from build123d import *

# Parameters (mm, degrees)
SKETCH_1_R          = 5.5
EXTRUDE_1_DEPTH     = 1
EXTRUDE_2_DEPTH     = 3
CUT_EXTRUDE_2_REACH = 8
SKETCH_9_R          = 2.5
CHAMFER_1_SIZE      = 0.3


with BuildPart() as part:
    # Эскиз1 → Бобышка-Вытянуть1 (new body)
    with BuildSketch(Plane.XY):
        Circle(SKETCH_1_R)
    extrude(amount=EXTRUDE_1_DEPTH)

    # Эскиз3 → Бобышка-Вытянуть2 (add)
    with BuildSketch(Plane.XY.offset(1)):
        Polygon((2.608163285, 3.811930956), (-1.997147402, 4.16470114), (-4.605310688, 0.352770185), (-2.608163285, -3.811930956), (1.997147402, -4.16470114), (4.605310688, -0.352770185), align=None)
    extrude(amount=EXTRUDE_2_DEPTH)

    # Эскиз5 → Вырез-Повернуть3 (revolve, cut)
    with BuildSketch(Plane(origin=(0, 0, 0), x_dir=(-0.997079012, 0.076376985, 0), z_dir=(-0.076376985, -0.997079012, 0))):
        Polygon((-4.618802154, -3.251492454), (-4.618802154, -4), (-3.987599163, -4), align=None)
    revolve(axis=Axis((0, 0, 0), (0, 0, 1)), mode=Mode.SUBTRACT)

    # Эскиз6 → Повернуть1 (revolve)
    with BuildSketch(Plane(origin=(0, 0, 0), x_dir=(0, 0, -1), z_dir=(1, 0, 0))):
        with BuildLine():
            Line((-4, 0), (-4, 3.75))
            ThreePointArc((-4, 3.75), (-5.062452688, 3.565118621), (-6, 3.032209738))
            Line((-6, 3.032209738), (-6, 0))
            Line((-6, 0), (-4, 0))
        make_face()
    revolve(axis=Axis((0, 0, 0.929807333), (0, 0, -1)))

    # Эскиз9 → Вырез-Вытянуть2 (cut, up to next)
    with BuildSketch(Plane(origin=(0, 0, 0), x_dir=(-1, 0, 0), z_dir=(0, 0, -1)), mode=Mode.PRIVATE) as cut_extrude_2_sk1:
        Circle(SKETCH_9_R)
    cut_extrude_2_tool1 = extrude(cut_extrude_2_sk1.sketch, amount=-CUT_EXTRUDE_2_REACH, mode=Mode.PRIVATE) & part.part
    add(cut_extrude_2_tool1.solids().sort_by_distance((0, 0, 0))[0], mode=Mode.SUBTRACT)

    # Фаска1
    chamfer_1_edges = [part.edges().sort_by_distance(p)[0] for p in [
        (2.5, 0, 0),
    ]]
    chamfer(chamfer_1_edges, length=CHAMFER_1_SIZE)


solid = part.part
Can you work these out from the model? Positions are in its coordinate system, mm. A direction names the side the tool comes from. Give positions to 0.01 mm unless a question says otherwise; leave off trailing zeros. Order: outer loops, then holes, each group sorted by start corner. A loop starts at its lowest first (then second) coordinate and runs counter-clockwise, first axis right, second up. Notation, with made-up numbers: M -14,27.5 L 34,27.5 A23 cw 34,64.5 Z; hole C 56.5,-23.5 d9. An arc over 180 degrees is marked long. One line per item, written item: value.
Item 1: Please list where these lines run through material, in increasing order: line 1 (X direction, y = 2, z = 4.5); line 2 (X direction, y = 0.25, z = 4.5); line 3 (Z direction, x = 3, y = -4.5).
Verdict:
line 1: -3.12 to -1.5, 1.5 to 3.12
line 2: -3.7 to -2.49, 2.49 to 3.7
line 3: 0 to 1
Item 2: If we mould it in two halves opening along X, with no side actions, what happens to faces 1 (the face through (-0.338, -3.986, 2.472)), 2 (the face through (1.2, 4.1, 1)), 3 (the face through (0.54, -2.44, 3.11))? For each: pulls with the +X half, pulls with the -X half, needs draft (parallel to the pull), parting line crosses it, or undercut.
Verdict:
face 1: pulls with the -X half
face 2: needs draft
face 3: undercut
Item 3: For faces 4 (the face through (3.28, -2.29, 2.47)), 5 (the face through (-3.28, 2.29, 2.47)), 6 (the face through (-3.62, -1.7, 2.47)), 7 (the face through (3.62, 1.7, 2.47)), which set-ups out of +Z, -Z, +X, -X, +Y, -Y let a thin tool reach every point of the face, with its end or its side?
Verdict:
face 4: +Z, +X, -Y
face 5: +Z, -X, +Y
face 6: +Z, -X, -Y
face 7: +Z, +X, +Y
Item 4: If we section it at A-A on z = 2: Write out the boundary of the cut face in (x, y), and give its area (3 significant figures).
Verdict:
outline: M -4.61,0.35 L -2.61,-3.81 L 2,-4.16 L 4.61,-0.35 L 2.61,3.81 L -2,4.16 Z; hole C 0,0 d5
area: 35.8 mm2
Item 5: If we section it at B-B on y = -4.5: Write out the boundary of the cut face in (x, z).
Verdict:
outline: M -3.16,0 L 3.16,0 L 3.16,1 L -3.16,1 Z
